The figure shows three views and two pictorial views of one solid part (mm, origin at its lowest corner). Answer the questions. A direction names the side the tool comes from. Coordinates: 2 decimals unless noted, no trailing zeros. Order: outer loops, then holes, each group sorted by start corner. A loop starts at its lowest first (then second) coordinate and runs counter-clockwise, first axis right, second up. Notation, with made-up numbers: M 33.5,25 L 57.5,25 A21 ccw 57.5,49 Z; hole C -31,-22 d1. An arc over 180 degrees is marked long. Use a Markdown table: item, result.
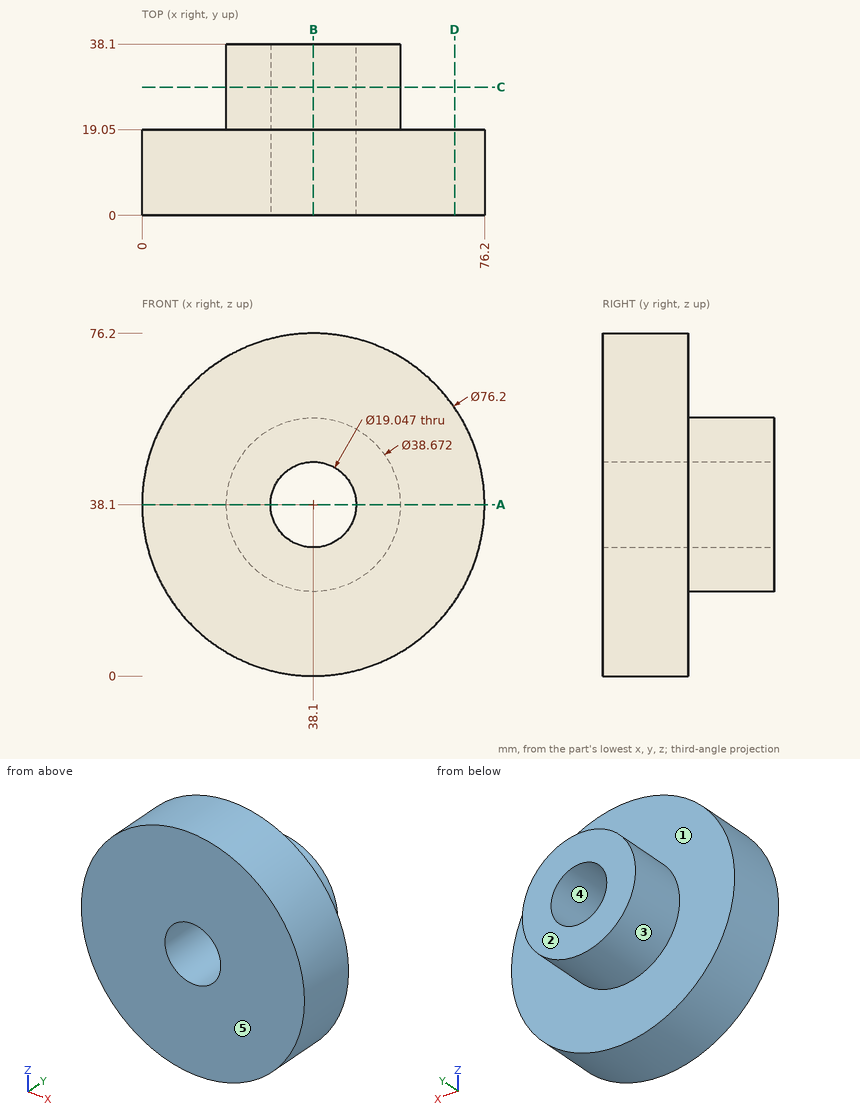
1. Flat-ended cylindrical pins translate along their axes: P1, Ø25, axis at x = 38.1, z = 38.1, coming from the -Y side; P2, Ø10, axis at y = 8, z = 22.5, coming from the -X side; P3, Ø6, axis at y = 9.5, z = 26, coming from the +X side; P4, Ø3, axis at x = 11.5, y = 15.5, coming from the +Z side. Find the tip coordinate at first contact, or state that the pin passes through.
Answers below:
| item | result |
|---|---|
| P1 | y = 0 |
| P2 | x = 1.5 |
| P3 | x = 75.1 |
| P4 | z = 66.76 |
2. Section B-B on x = 38.1 is taken. Determine the outline of the cut face in (y, z), then the cut area to 3 significant figures.
Answers below:
| item | result |
|---|---|
| outline | M 0,0 L 19.05,0 L 19.05,18.76 L 38.1,18.76 L 38.1,28.58 L 0,28.58 Z; M 0,47.62 L 38.1,47.62 L 38.1,57.44 L 19.05,57.44 L 19.05,76.2 L 0,76.2 Z |
| area | 1,460 mm² |
3. Find the intervals of material crossed by probe 1 along Z at (x, y) = (38.1, 24); probe 2 along Y at (x, z) = (60, 26.5); probe 3 along X at (y, z) = (33, 39.5), in increasing order.
Answers below:
| item | result |
|---|---|
| probe 1 | 18.76 to 28.58, 47.62 to 57.44 |
| probe 2 | 0 to 19.05 |
| probe 3 | 18.81 to 28.68, 47.52 to 57.39 |
4. Section A-A on z = 38.1 is taken. Determine the outline of the cut face in (x, y).
Answers below:
| item | result |
|---|---|
| outline | M 0,0 L 28.58,0 L 28.58,38.1 L 18.76,38.1 L 18.76,19.05 L 0,19.05 Z; M 47.62,0 L 76.2,0 L 76.2,19.05 L 57.44,19.05 L 57.44,38.1 L 47.62,38.1 Z |
5. For a pull along X with two mould halves and no side action, classify the marked faces 3, 4 and 5 as +X half, -X half, draft (parallel to the pull), parting line (faces both ways), or undercut.
Answers below:
| item | result |
|---|---|
| face 3 | parting line |
| face 4 | undercut |
| face 5 | draft |
6. For the marked faces 1 and 2, determine the directions among +Z, -Z, +X, -X, +Y, -Y from which every point of the face is accessible in a straight line to the end or side of a thin tool.
Answers below:
| item | result |
|---|---|
| face 1 | +Y |
| face 2 | +Z, -Z, +X, -X, +Y |
7. Section C-C on y = 28.5 is taken. Determine the outline of the cut face in (x, z).
Answers below:
| item | result |
|---|---|
| outline | C 38.1,38.1 d38.67; hole C 38.1,38.1 d19.05 |
8. Section D-D on x = 69.5 is taken. Determine the outline of the cut face in (y, z).
Answers below:
| item | result |
|---|---|
| outline | M 0,16.52 L 19.05,16.52 L 19.05,59.68 L 0,59.68 Z |
